Work out the finished part from the listing and answer in its coordinate system (mm). A direction names the side the tool comes from. Give positions to 0.01 mm unless a question says otherwise; leave off trailing zeros. Loops run counter-clockwise (first coordinate to the right, second up) from the corner with the lowest first, then second, coordinate; pieces in that order, holes last. Notation, with made-up numbers: M 9.25,75.5 L 64.25,75.5 A26 cw 64.25,106.5 Z; hole C 21.5,45.5 d5. An arc over 180 degrees is marked long. Use a Markdown table: item, result.
Autodesk Inventor part; units mm, degrees
ref_plane "YZ Plane" through (0, 0, 0) normal (1, 0, 0) x (0, 1, 0)
ref_plane "XZ Plane" through (0, 0, 0) normal (0, 1, 0) x (-1, 0, 0)
ref_plane "XY Plane" through (0, 0, 0) normal (0, 0, 1) x (1, 0, 0)
sketch "Sketch1" plane through (0, 0, 0) normal (0, 0, 1) x (1, 0, 0)
  circle A0 centre (0, 0) radius 5.25
  circle A1 centre (0, 0) radius 6.825
  dimension "d0" = 10.5
  dimension "d1" = 13.65
extrude "Extrusion1" add sketch "Sketch1" along normal blind 4
extrude "Extrusion2" add sketch "Sketch1" against normal blind 6 contours A0 | A1
sketch "Sketch2" plane through (0, 0, -6) normal (0, 0, -1) x (-1, 0, 0)
  circle A0 centre (0, 0) radius 3.5
  line L0 (-2.1, 2.8) -> (2.1, 2.8)
  dimension "d6" = 7
  dimension "d7" = 0.7
extrude "Extrusion3" cut sketch "Sketch2" against normal blind 4 contours A0 L0 picked at (-0.6426, 0.8929)
properties part number "Shaft Coupler"
(1) Consider probe 1 along Y at (x, z) = (0, -4.95) (3 decimals); probe 2 along Y at (x, z) = (0, 2) (3 decimals); probe 3 along Z at (x, y) = (-0.5, -2). Determine where each line is inside the solid, lowest interval first. Write a range as [from, to].
Entries:
| item | result |
|---|---|
| probe 1 | y = [-6.825, -3.5], [2.8, 6.825] |
| probe 2 | y = [-6.825, -5.25], [5.25, 6.825] |
| probe 3 | z = [-2, 0] |
(2) A cutting plane is placed at D-D (z = -1.25). Write down the section's boundary in (x, y) (3 decimals), and give its area (3 significant figures).
Entries:
| item | result |
|---|---|
| outline | C 0,0 d13.65 |
| area | 146 mm² |
(3) A cutting plane is placed at A-A (y = 0). Write down the section's boundary in (x, z) (3 decimals), and give its area (3 significant figures).
Entries:
| item | result |
|---|---|
| outline | M -6.825,-6 L -3.5,-6 L -3.5,-2 L 3.5,-2 L 3.5,-6 L 6.825,-6 L 6.825,4 L 5.25,4 L 5.25,0 L -5.25,0 L -5.25,4 L -6.825,4 Z |
| area | 66.5 mm² |
(4) A cutting plane is placed at B-B (x = 0). Write down the section's boundary in (y, z) (3 decimals).
Entries:
| item | result |
|---|---|
| outline | M -6.825,-6 L -3.5,-6 L -3.5,-2 L 2.8,-2 L 2.8,-6 L 6.825,-6 L 6.825,4 L 5.25,4 L 5.25,0 L -5.25,0 L -5.25,4 L -6.825,4 Z |
(5) A cutting plane is placed at C-C (z = 3). Write down the section's boundary in (x, y) (3 decimals).
Entries:
| item | result |
|---|---|
| outline | C 0,0 d13.65; hole C 0,0 d10.5 |
(6) Given P1, Ø4, axis at y = -3.5, z = 0, coming from the +X side; P2, Ø1, axis at x = 1.5, y = -4, coming from the +Z side; P3, Ø3, axis at x = -1.5, y = 0, coming from the -Z side; P4, Ø6.5, axis at x = 0, y = 0, coming from the -Z side, each flat-ended and moving along its own axis, determine where each tip first touches the part or whether it passes through.
Entries:
| item | result |
|---|---|
| P1 | stops at x = 6.66 |
| P2 | stops at z = 0 |
| P3 | stops at z = -2 |
| P4 | stops at z = -6 |
(7) Which of the six approach directions +Z, -Z, +X, -X, +Y, -Y give full straight-line access (tool end or side, diameter ignored) to faces 4 (the cylindrical face through (5, -1.6, 2)), 5 (the cylindrical face through (0.1, -3.5, -4)), 6 (the flat face through (0, 3, -6))?
Entries:
| item | result |
|---|---|
| face 4 | +Z |
| face 5 | -Z |
| face 6 | -Z, +X, -X, +Y, -Y |
(8) The mould has two halves that part along Y. Classify faces 1 (the flat face through (4, -4, 4)), 2 (the cylindrical face through (-5.42, -4.15, -0.93)), 3 (the flat face through (0, 0, -2)): released by +Y, released by -Y, zero draft, split by the parting line, or undercut.
Entries:
| item | result |
|---|---|
| face 1 | zero draft |
| face 2 | split by the parting line |
| face 3 | undercut |
